For this review, take the finished solid that the model builds, in its own axes (mm). A direction names the side the tool comes from. Give positions to 0.01 mm unless a question says otherwise; leave off trailing zeros. Write each loop counter-clockwise with the first axis right and the second up, starting at its lowest first coordinate (ties: lowest second). Pieces come first, ordered by that corner, then holes. Notation, with made-up numbers: (80, 18) -> (110, 18) arc R25 cw to (110, 51) -> close; hole circle Ø10 at (7, 9.25). An arc over 180 degrees is marked (long way). Answer as CSV lines item,"result".
Autodesk Inventor part; units mm, degrees
ref_plane "YZ Plane" through (0, 0, 0) normal (1, 0, 0) x (0, 1, 0)
ref_plane "XZ Plane" through (0, 0, 0) normal (0, 1, 0) x (-1, 0, 0)
ref_plane "XY Plane" through (0, 0, 0) normal (0, 0, 1) x (1, 0, 0)
sketch "スケッチ1" plane through (0, 0, 0) normal (0, 0, 1) x (1, 0, 0)
  line L0 (-29.15, 14.5) -> (29.15, 14.5)
  line L1 (29.15, 14.5) -> (29.15, -14.5)
  line L2 (29.15, -14.5) -> (-29.15, -14.5)
  line L3 (-29.15, -14.5) -> (-29.15, 14.5)
  line L4 (-24.15, 11.5) -> (24.15, 11.5) construction
  line L5 (24.15, 11.5) -> (24.15, -11.5) construction
  line L6 (24.15, -11.5) -> (-24.15, -11.5) construction
  line L7 (-24.15, -11.5) -> (-24.15, 11.5) construction
  line L8 (24.15, 11.5) -> (-24.15, -11.5) construction
  line L9 (-24.15, -9.8386) -> (-24.15, 11.5)
  line L10 (-24.15, 11.5) -> (20.6611, 11.5)
  line L11 (20.6611, 11.5) -> (-24.15, -9.8386)
  line L12 (-20.6611, -11.5) -> (24.15, -11.5)
  line L13 (24.15, -11.5) -> (24.15, 9.8386)
  line L14 (24.15, 9.8386) -> (-20.6611, -11.5)
  line L15 (-29.15, 12) -> (29.15, 12) construction
  line L16 (29.15, -12) -> (-29.15, -12) construction
  line L17 (29.15, 12) -> (29.15, -12) construction
  point P0 (0, 0)
  point P1 (0, 11.5)
  point P2 (0, 14.5)
  point P3 (24.15, 0)
  point P4 (29.15, 0)
  dimension "d0" = 5
  dimension "d1" = 3
  dimension "d2" = 1.5
  dimension "d3" = 24
  dimension "d4" = 2.5
  dimension "d16" = 58.3
extrude "押し出し1" add sketch "スケッチ1" along normal blind 5
sketch "スケッチ2" plane through (29.15, -14.5, 0) normal (1, 0, 0) x (0, 0, -1)
  line L0 (0, 29) -> (-5, 29)
  line L1 (-5, 0) -> (-5, 29)
  line L2 (0, 14.5) -> (-5, 14.5) construction
  point P0 (-2.5, 2.5)
  point P1 (-2.5, 14.5)
  point P2 (-2.5, 26.5)
  point P3 (-2.5, 29)
  dimension "d7" = 24
hole "穴1" at (29.15, -12, 2.5) at (29.15, 0, 2.5) at (29.15, 12, 2.5) direction (-1, 0, 0) diameter 2.459 depth 3
mirror "ミラー1" about plane through (0, 0, 0) normal (1, 0, 0) of "穴1"
fillet "フィレット1" radius 2 6 edges at (-20.6611, -11.5, 2.5) (-24.15, -9.8386, 2.5) (24.15, 9.8386, 2.5) (24.15, -11.5, 2.5) (-24.15, 11.5, 2.5) (20.6611, 11.5, 2.5)
equation "\"d3\" = d5_1"
properties part number "リンク_ふくらはぎ_サブフレーム_1_2(予備案)" material "アルミニウム 2014-T4"
Q1. Draft analysis for pull direction Z (two halves, no side actions). For faces 6 (the cylindrical face through (27.629, 11.631, 1.327)), 7 (the flat face through (4.548, 0.504, 2.465)), 8 (the flat face through (0, 0, 0)), state which applies: released by +Z, released by -Z, zero draft, split by the parting line, or undercut.
Answer block:
face 6,"undercut"
face 7,"zero draft"
face 8,"released by -Z"
Q2. Clearance check with flat-ended pins moving along their axes: pin 1 (2 mm diameter, centred on y = -12, z = 2, fed in from +X); pin 2 (2 mm diameter, centred on y = 0, z = 2.5, fed in from +X); pin 3 (2 mm diameter, centred on y = 12, z = 2.5, fed in from -X). State where each tip first meets the part, or that it passes through.
Answer block:
pin 1,"stops at x = 29.15"
pin 2,"stops at x = 26.15"
pin 3,"stops at x = -26.15"
Q3. Add section B-B (y = 0). Write out the cut boundary in (x, z).
Answer block:
outline,"(-29.15, 0) -> (-24.15, 0) -> (-24.15, 5) -> (-29.15, 5) -> (-29.15, 3.73) -> (-26.15, 3.73) -> (-26.15, 1.27) -> (-29.15, 1.27) -> close; (-3.49, 0) -> (3.49, 0) -> (3.49, 5) -> (-3.49, 5) -> close; (24.15, 0) -> (29.15, 0) -> (29.15, 1.27) -> (26.15, 1.27) -> (26.15, 3.73) -> (29.15, 3.73) -> (29.15, 5) -> (24.15, 5) -> close"
Q4. Add section C-C (z = 2.5). State how many separate pieces and enclosed holes the cut face has, plus the area to 3 significant figures.
Answer block:
separate pieces,"1"
enclosed holes,"2"
area,"721 mm2"
Q5. Add section D-D (y = -5). Write out the cut boundary in (x, z).
Answer block:
outline,"(-29.15, 0) -> (-24.15, 0) -> (-24.15, 5) -> (-29.15, 5) -> close; (-13.99, 0) -> (-7.01, 0) -> (-7.01, 5) -> (-13.99, 5) -> close; (24.15, 0) -> (29.15, 0) -> (29.15, 5) -> (24.15, 5) -> close"
Q6. Add section A-A (x = -1). Write out the cut boundary in (y, z).
Answer block:
outline,"(-14.5, 0) -> (-11.5, 0) -> (-11.5, 5) -> (-14.5, 5) -> close; (-2.14, 0) -> (1.19, 0) -> (1.19, 5) -> (-2.14, 5) -> close; (11.5, 0) -> (14.5, 0) -> (14.5, 5) -> (11.5, 5) -> close"
Q7. For faces 1 (the cylindrical face through (-27.629, -11.631, 1.327)), 2 (the flat face through (-5, 11.5, 2)), 3 (the flat face through (26.15, 0, 3)), 4 (the flat face through (-29.15, 0, 1)), 5 (the flat face through (0, 14.5, 2)), list the 3-axis set-ups (+Z, -Z, +X, -X, +Y, -Y) from which the entire face can be reached by the end or side of a thin tool; tool diameter is ignored.
Answer block:
face 1,"-X"
face 2,"+Z, -Z"
face 3,"+X"
face 4,"+Z, -Z, -X, +Y, -Y"
face 5,"+Z, -Z, +X, -X, +Y"
Q8. To check wall thickness, follow probe 1 along Z at (x, y) = (27.9, 0); probe 2 along Y at (x, z) = (-27.5, 2.5); probe 3 along X at (y, z) = (3, 2.6). State the ranges of each line that lie inside material, in increasing order. Write a range as [from, to].
Answer block:
probe 1,"z = [0, 1.27], [3.73, 5]"
probe 2,"y = [-14.5, -13.23], [-10.77, -1.23], [1.23, 10.77], [13.23, 14.5]"
probe 3,"x = [-29.15, -24.15], [2.81, 9.79], [24.15, 29.15]"
